from build123d import *

# Parameters (mm, degrees)
F1_DEPTH = 1.75
F2_R     = 21.5
F3_DEPTH = 25
F4_R     = 21.5
F5_DEPTH = 15


with BuildPart() as f1:
    # F0 (on Front) → F1 (new body)
    with BuildSketch(Plane.XZ):
        Polygon((75.75, 0), (0, 0), (0, -48), (4, -48), (4, -50), (71.75, -50), (71.75, -48), (75.75, -48), align=None)
    extrude(amount=F1_DEPTH)

    # F2 (on face) → F3 (cut)
    with BuildSketch(Plane.XZ.offset(1.75)):
        with Locations((37.875, -27.5)):
            Circle(F2_R)
    extrude(amount=-F3_DEPTH, mode=Mode.SUBTRACT)

    # F4 (on face) → F5 (join)
    with BuildSketch(Plane.XZ.offset(1.75)):
        with BuildLine():
            ThreePointArc((37.875, -50), (53.7849025767, -43.4099025767), (60.375, -27.5))
            ThreePointArc((60.375, -27.5), (21.9650974233, -11.5900974233), (37.875, -50))
        make_face()
        with Locations((37.875, -27.5)):
            Circle(F4_R, mode=Mode.SUBTRACT)
    extrude(amount=F5_DEPTH)


solid = f1.part
Geometry: final body of the model. Coordinates: model frame, mm. A direction names the side the tool comes from. Round coordinates to 2 decimals unless told otherwise and drop trailing zeros. Loops run counter-clockwise (first coordinate to the right, second up) from the corner with the lowest first, then second, coordinate; pieces in that order, holes last. Notation, with made-up numbers: (-7.5, 76.5) - (45.5, 76.5) arc R20 ccw to (45.5, 100.5) - close; hole circle Ø2 at (27.5, 52). An arc over 180 degrees is marked (long way). Write each question's results on one line, items separated by ' | '. Start each with the question number.
1) Cut plane C-C on y = -10.5. Return loops of the section in (x, z) (3 decimals).
2) Cut plane A-A on z = -27.5. Return loops of the section in (x, y) (3 decimals), then the cut area to 3 significant figures.
3) Cut plane B-B on x = 51.5. Return loops of the section in (y, z).
4) Access query for faces 4 (the face through (75.75, -1, -24)), 5 (the face through (59.336, -9.145, -20.742)), 6 (the face through (2, -1, -48)), 7 (the face through (71.75, -1, -49)). Directions: +Z, -Z, +X, -X, +Y, -Y. A direction counts if a zero-diameter tool reaches every point of the face in a straight line with its end or side. Return the directions, or none.
5) Line query: probe 1 along Y at (x, z) = (53, -8.5); probe 2 along X at (y, z) = (-9.25, -12); probe 3 along X at (y, z) = (-10.25, -20.5). Output: solid intervals per line, ascending. Write a range as [from, to].
6) First-contact query: P1, Ø1.5, axis at y = -6.5, z = -44, coming from the -X side; P2, Ø3, axis at x = 43, y = -3.5, coming from the -Z side; P3, Ø0.5, axis at x = 74, y = -0.5, coming from the -Z side. Flat tips, straight axial feed; report the tip coordinate or a pass-through.
7) Mould query, pull axis Y, two halves, no side actions, for faces 1 (the face through (37, -1.75, -2)), 2 (the face through (20.5, 0, -13.5)), 3 (the face through (74, -1, -48)). Classes: released by +Y, released by -Y, zero draft, split by the parting line, or undercut.
8) Cut plane D-D on x = 14. Return loops of the section in (y, z).
Verdict:
1) outline: circle Ø45 at (37.875, -27.5); hole circle Ø43 at (37.875, -27.5)
2) outline: (0, -1.75) - (15.375, -1.75) - (15.375, -16.75) - (16.375, -16.75) - (16.375, 0) - (0, 0) - close; (59.375, -16.75) - (60.375, -16.75) - (60.375, -1.75) - (75.75, -1.75) - (75.75, 0) - (59.375, 0) - close | area: 87.3 mm2
3) outline: (-16.75, -45.41) - (-1.75, -45.41) - (-1.75, -50) - (0, -50) - (0, -44.13) - (-16.75, -44.13) - close; (-16.75, -10.87) - (0, -10.87) - (0, 0) - (-1.75, 0) - (-1.75, -9.59) - (-16.75, -9.59) - close
4) face 4: +Z, -Z, +X, +Y, -Y | face 5: -Y | face 6: -Z, -X, +Y, -Y | face 7: -Z, +X, +Y, -Y
5) probe 1: y = [-1.75, 0] | probe 2: x = [21.57, 22.98], [52.77, 54.18] | probe 3: x = [16.49, 17.55], [58.2, 59.26]
6) P1: stops at x = 21.81 | P2: stops at z = -49.71 | P3: stops at z = -48
7) face 1: released by -Y | face 2: released by +Y | face 3: zero draft
8) outline: (-1.75, -50) - (0, -50) - (0, 0) - (-1.75, 0) - close
